Drawing for the job (mm, zero at the part's lowest x, y, z). Round coordinates to 2 decimals unless told otherwise and drop trailing zeros. Write each loop counter-clockwise with the first axis right and the second up, starting at its lowest first coordinate (ties: lowest second). Pieces come first, ordered by that corner, then holes.
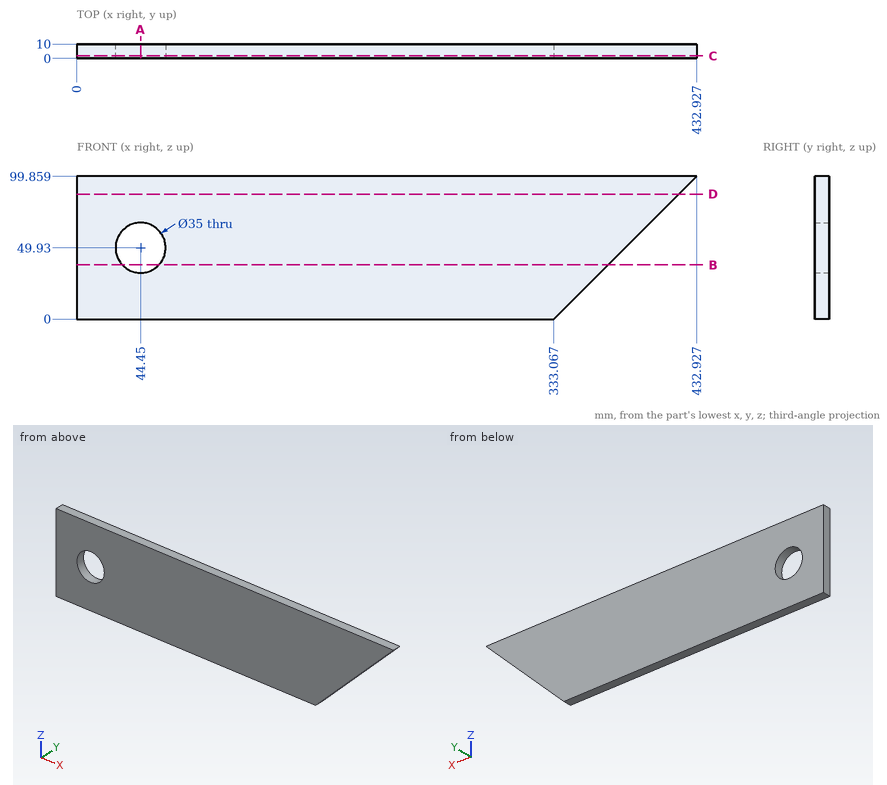
1) Flat gauge pins, fed straight in: pin 1 Ø3 at (y, z) = (8.5, 84.5) entering from +X; pin 2 Ø3 at (y, z) = (6.5, 80) entering from +X. Where does each tip first touch, or does it go through?
2) Cut at B-B on z = 38. List the corners of the cut face in (x, y).
3) Cut at A-A on x = 44.45. List the corners of the cut face in (y, z).
4) Wall check: probe 1 along Z at (x, y) = (44.45, 2.75); probe 2 along X at (y, z) = (0.75, 48.5) (1 decimal); probe 3 along X at (y, z) = (5.5, 38) (1 decimal). Give the ranges that are in metal, low to high.
5) Cut at D-D on z = 87.5. List the corners of the cut face in (x, y).
6) Cut at C-C on y = 1.75. List the corners of the cut face in (x, z), and give its area (3 significant figures).
Result sheet:
1. pin 1: stops at x = 419.07
1. pin 2: stops at x = 414.57
2. outline: (0, 0) - (31.65, 0) - (31.65, 10) - (0, 10) - close; (57.25, 0) - (371.07, 0) - (371.07, 10) - (57.25, 10) - close
3. outline: (0, 0) - (10, 0) - (10, 32.43) - (0, 32.43) - close; (0, 67.43) - (10, 67.43) - (10, 99.86) - (0, 99.86) - close
4. probe 1: z = 0 to 32.43, 67.43 to 99.86
4. probe 2: x = 0 to 27, 61.9 to 381.6
4. probe 3: x = 0 to 31.6, 57.3 to 371.1
5. outline: (0, 0) - (420.57, 0) - (420.57, 10) - (0, 10) - close
6. outline: (0, 0) - (333.07, 0) - (432.93, 99.86) - (0, 99.86) - close; hole circle Ø35 at (44.45, 49.93)
6. area: 37,300 mm2
